Geometry check sheet. Reference: drawing and pictorial views, mm from the part's lowest x, y, z. A direction names the side the tool comes from. Coordinates: 2 decimals unless noted, no trailing zeros. Loops run counter-clockwise (first coordinate to the right, second up) from the corner with the lowest first, then second, coordinate; pieces in that order, holes last. Notation, with made-up numbers: (47.5, 47) -> (96.5, 47) arc R23 cw to (96.5, 64) -> close; hole circle Ø1 at (18, 23.25). An arc over 180 degrees is marked (long way). Answer as a JSON object with one key per item and string values.
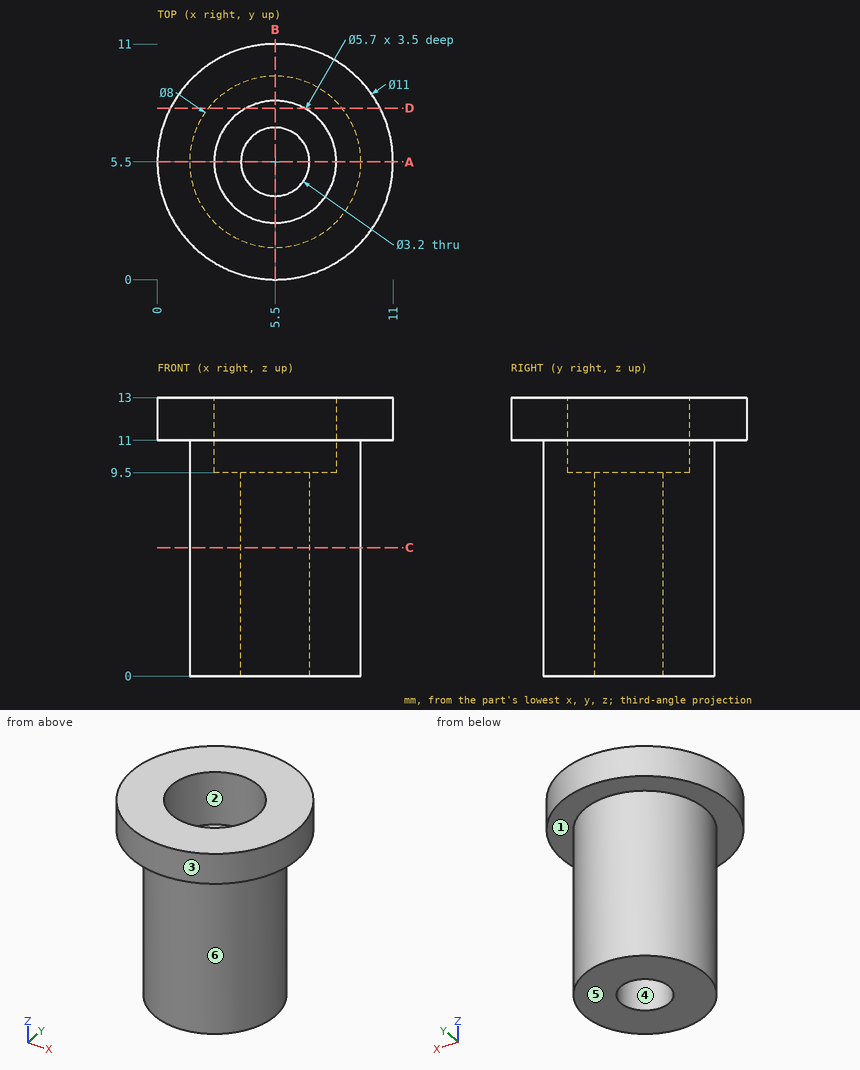
1. Tool access check on the marked faces 5 and 6. Record the directions out of +Z, -Z, +X, -X, +Y, -Y that give a thin tool (end or side, any length) a straight path to the whole face; none if there is none.
Evaluation:
{"face 5": "-Z, +X, -X, +Y, -Y", "face 6": "-Z"}
2. Depth check by flat-ended pin: P1, Ø1.5, axis at y = 5, z = 10.5, coming from the +X side; P2, Ø4, axis at x = 1.5, z = 3, coming from the +Y side; P3, Ø4, axis at x = 9, z = 8.5, coming from the -Y side; P4, Ø3, axis at x = 4.5, y = 6, coming from the +Z side. Enter the tip coordinate at first touch or a pass-through.
Evaluation:
{"P1": "stops at x = 11", "P2": "stops at y = 8.96", "P3": "stops at y = 1.79", "P4": "stops at z = 9.5"}
3. Section check C-C, the plane z = 6. Record the boundary of the cut face in (x, y), then the cut area to 3 significant figures.
Evaluation:
{"outline": "circle Ø8 at (5.5, 5.5); hole circle Ø3.2 at (5.5, 5.5)", "area": "42.2 mm^2"}
4. Thickness scan on probe 1 along Y at (x, z) = (5.5, 1.5); probe 2 along Y at (x, z) = (5.5, 10.5); probe 3 along Z at (x, y) = (8, 6.75). Record the ranges inside material, lowest first. Write a range as from..to.
Evaluation:
{"probe 1": "y = 1.5..3.9, 7.1..9.5", "probe 2": "y = 1.5..2.65, 8.35..9.5", "probe 3": "z = 0..9.5"}
5. Section check D-D, the plane y = 8. Record the boundary of the cut face in (x, z), then the cut area to 3 significant figures.
Evaluation:
{"outline": "(0.6, 11) -> (2.38, 11) -> (2.38, 0) -> (8.62, 0) -> (8.62, 11) -> (10.4, 11) -> (10.4, 13) -> (6.87, 13) -> (6.87, 9.5) -> (4.13, 9.5) -> (4.13, 13) -> (0.6, 13) -> close", "area": "78.7 mm^2"}
6. Section check A-A, the plane y = 5.5. Record the boundary of the cut face in (x, z), then the cut area to 4 significant figures.
Evaluation:
{"outline": "(0, 11) -> (1.5, 11) -> (1.5, 0) -> (3.9, 0) -> (3.9, 9.5) -> (2.65, 9.5) -> (2.65, 13) -> (0, 13) -> close; (7.1, 0) -> (9.5, 0) -> (9.5, 11) -> (11, 11) -> (11, 13) -> (8.35, 13) -> (8.35, 9.5) -> (7.1, 9.5) -> close", "area": "59.65 mm^2"}
7. Mould release check, pull along X, two halves, no side actions. Record for the marked faces 1, 2, 3 and 4: released by +X, released by -X, zero draft, split by the parting line, or undercut.
Evaluation:
{"face 1": "zero draft", "face 2": "undercut", "face 3": "split by the parting line", "face 4": "undercut"}
